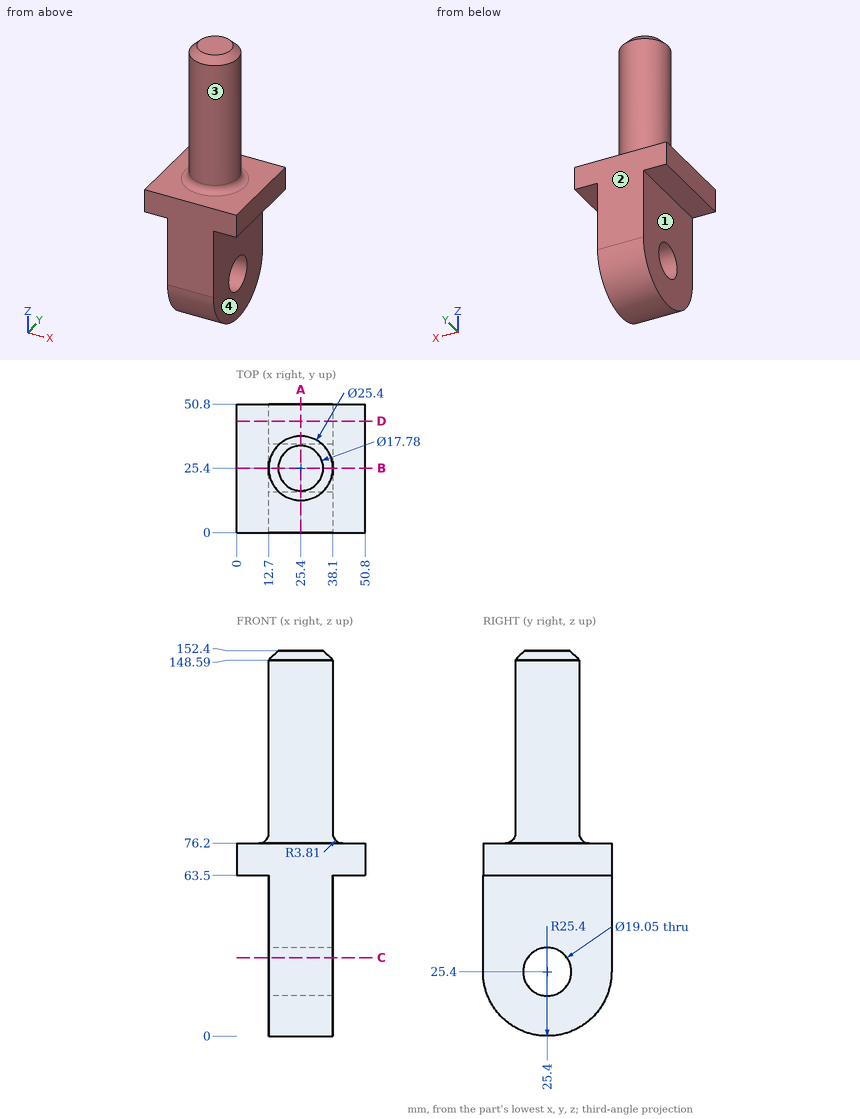
The drawing under review shows one solid part. Ordinate dimensions are in mm from its lowest x, y, z. A direction names the side the tool comes from. Coordinates: 2 decimals unless noted, no trailing zeros. Write each loop counter-clockwise with the first axis right and the second up, starting at its lowest first coordinate (ties: lowest second). Pieces come first, ordered by that corner, then holes.
1) Add section C-C (z = 31). Write out the cut boundary in (x, y).
2) To check wall thickness, follow L1, parallel to Y at x = 28, z = 25; L2, parallel to Z at x = 25, y = 25; L3, parallel to Y at x = 21, z = 32. State the ranges of each line that lie inside material, in increasing order.
3) Machinability: for the marked faces 1, 2, 3 and 4, which of the approach directions +Z, -Z, +X, -X, +Y, -Y give a long, thin tool a straight path to every point of the face, cutting with its end or side? Answer none if there is none.
4) Add section D-D (y = 44). Write out the cut boundary in (x, z), plus the area to 3 significant figures.
5) Add section B-B (y = 25.4). Write out the cut boundary in (x, z) (3 decimals).
6) Add section A-A (x = 25.4). Write out the cut boundary in (y, z) (3 decimals), plus the area to 3 significant figures.
7) Insertion check: pin 1 (14 mm diameter, centred on x = 41.5, y = 18, fed in from -Z); pin 2 (8 mm diameter, centred on x = 23.5, y = 5.5, fed in from +Z); pin 3 (3 mm diameter, centred on y = 17, z = 34, fed in from +X); pin 4 (17 mm diameter, centred on y = 25.4, z = 25.4, fed in from -X). Each pin has a flat end and moves straight along its axis. Give the tip position at first contact, or say it passes through.
Check result:
1. outline: (12.7, 0) - (38.1, 0) - (38.1, 17.7) - (12.7, 17.7) - close; (12.7, 33.1) - (38.1, 33.1) - (38.1, 50.8) - (12.7, 50.8) - close
2. L1: y = 0 to 15.88, 34.92 to 50.8
2. L2: z = 0 to 15.88, 34.92 to 152.4
2. L3: y = 0 to 18.53, 32.27 to 50.8
3. face 1: -Z, -X, +Y, -Y
3. face 2: +Z, -Z, +X, -X, +Y
3. face 3: +Z
3. face 4: -Z, +X, +Y, -Y
4. outline: (0, 63.5) - (12.7, 63.5) - (12.7, 8.1) - (38.1, 8.1) - (38.1, 63.5) - (50.8, 63.5) - (50.8, 76.2) - (0, 76.2) - close
4. area: 2,050 mm2
5. outline: (0, 63.5) - (12.7, 63.5) - (12.7, 34.925) - (38.1, 34.925) - (38.1, 63.5) - (50.8, 63.5) - (50.8, 76.2) - (41.91, 76.2) arc R3.81 cw to (38.1, 80.01) - (38.1, 148.59) - (34.29, 152.4) - (16.51, 152.4) - (12.7, 148.59) - (12.7, 80.01) arc R3.81 cw to (8.89, 76.2) - (0, 76.2) - close; (12.7, 0) - (38.1, 0) - (38.1, 15.875) - (12.7, 15.875) - close
6. outline: (0, 25.4) arc R25.4 ccw to (50.8, 25.4) - (50.8, 76.2) - (41.91, 76.2) arc R3.81 cw to (38.1, 80.01) - (38.1, 148.59) - (34.29, 152.4) - (16.51, 152.4) - (12.7, 148.59) - (12.7, 80.01) arc R3.81 cw to (8.89, 76.2) - (0, 76.2) - close; hole circle Ø19.05 at (25.4, 25.4)
6. area: 5,240 mm2
7. pin 1: stops at z = 0.03
7. pin 2: stops at z = 76.24
7. pin 3: stops at x = 38.1
7. pin 4: passes through
